```python
from build123d import *

# Parameters (mm, degrees)
BOSS_EXTRUDE1_DEPTH       = 25
F_1_0MM_DOWEL_HOLE1_D     = 10
F_1_0MM_DOWEL_HOLE1_DEPTH = 25
M8X1_0_TAPPED_HOLE1_D     = 7
M8X1_0_TAPPED_HOLE1_DEPTH = 15


# Read off the part's stored shape, not the designer's step: CSK for M6 Flat Head Machine Screw1
with BuildPart() as part:
    # Sketch1 → Boss-Extrude1 (new, symmetric)
    with BuildSketch(Plane.XY):
        Polygon((0, 0), (0, 97), (-45, 97), (-45, 84), (-39, 84), (-39, 90), (-32, 90), (-32, 0), align=None)
    extrude(amount=BOSS_EXTRUDE1_DEPTH, both=True)

    # Ø1.0mm Dowel Hole1
    with Locations(Plane.XY.offset(25)):
        with Locations((-16, 45)):
            Hole(F_1_0MM_DOWEL_HOLE1_D / 2, depth=F_1_0MM_DOWEL_HOLE1_DEPTH)

    # M8x1.0 Tapped Hole1
    with Locations(Plane(origin=(0, 0, 0), x_dir=(-1, 0, 0), z_dir=(0, -1, 0))):
        with Locations((7, 0), (25, 0)):
            Hole(M8X1_0_TAPPED_HOLE1_D / 2, depth=M8X1_0_TAPPED_HOLE1_DEPTH)

    # CSK for M6 Flat Head Machine Screw1 outl → CSK for M6 Flat Head Machine Screw1 (revolve, cut)
    with BuildSketch(Plane(origin=(0, 45, 9), x_dir=(0, 1, 0), z_dir=(0, 0, -1))):
        Polygon((0, -12.244302381), (3.3, -12.244302381), (3.3, -3), (6.3, 0), (0, 0), align=None)
    revolve(axis=Axis((0, 45, 9), (1, 0, 0)), mode=Mode.SUBTRACT)


solid = part.part
```
For this review, take the finished solid that the model builds, in its own axes (mm). A direction names the side the tool comes from. Round coordinates to 2 decimals unless told otherwise and drop trailing zeros. Write each loop counter-clockwise with the first axis right and the second up, starting at its lowest first coordinate (ties: lowest second). Pieces come first, ordered by that corner, then holes.
1) Mouldability with a two-part tool opening along Z and no side actions: class faces 1 (the face through (-25, 15, 0)), 2 (the face through (-16, 45, 0)), 3 (the face through (-7, 15, 0)), 4 (the face through (-32, 46, 0)) as +Z half, -Z half, draft (parallel to the pull), parting line (faces both ways), or undercut.
Answer below:
face 1: undercut
face 2: +Z half
face 3: undercut
face 4: draft
2) Take a section at A-A on y = 45. Give the boundary of the cut face in (x, z), then the cut area to 3 significant figures.
Answer below:
outline: (-32, -25) - (0, -25) - (0, 2.7) - (-3, 5.7) - (-11, 5.7) - (-11, 0) - (-21, 0) - (-21, 25) - (-32, 25) - close; (-11, 12.3) - (-3, 12.3) - (0, 15.3) - (0, 25) - (-11, 25) - close
area: 1,270 mm2
3) Insertion check: pin 1 Ø7.5 at (x, z) = (-36.5, 8.5) entering from -Y; pin 2 Ø3 at (y, z) = (68, 10.5) entering from -X; pin 3 Ø2 at (x, z) = (-25, 0) entering from -Y; pin 4 Ø6 at (x, y) = (-36.5, 73.5) entering from +Z. Each pin has a flat end and moves straight along its axis. Give the tip position at first contact, or say it passes through.
Answer below:
pin 1: stops at y = 84
pin 2: stops at x = -32
pin 3: stops at y = 15
pin 4: passes through
4) Take a section at B-B on x = -7. Give the boundary of the cut face in (y, z), then the cut area to 3 significant figures.
Answer below:
outline: (0, -25) - (97, -25) - (97, 25) - (0, 25) - (0, 3.5) - (15, 3.5) - (15, -3.5) - (0, -3.5) - close; hole circle Ø6.6 at (45, 9)
area: 4,710 mm2
5) Take a section at D-D on x = -19.5. Give the boundary of the cut face in (y, z), then the cut area to 3 significant figures.
Answer below:
outline: (0, -25) - (97, -25) - (97, 25) - (48.57, 25) - (48.57, 0) - (41.43, 0) - (41.43, 25) - (0, 25) - close
area: 4,670 mm2
6) Take a section at C-C on z = -15.5. Give the boundary of the cut face in (x, y).
Answer below:
outline: (-45, 84) - (-39, 84) - (-39, 90) - (-32, 90) - (-32, 0) - (0, 0) - (0, 97) - (-45, 97) - close
7) For line 1 along Z through (x, y) = (-9, 45); line 2 along Z through (x, y) = (-7, 9); line 3 along Y through (x, z) = (-5, 9), list the stretches that pass through material, from the lowest coordinate up.
Answer below:
line 1: z = -25 to 5.7, 12.3 to 25
line 2: z = -25 to -3.5, 3.5 to 25
line 3: y = 0 to 41.7, 48.3 to 97
8) Machinability: for faces 5 (the face through (-39, 87, 0)), 6 (the face through (-42, 84, 0)), 7 (the face through (-10.497, 7.605, -0.154)), 8 (the face through (-7.56, 44.28, 5.78)), which of the approach directions +Z, -Z, +X, -X, +Y, -Y give a long, thin tool a straight path to every point of the face, cutting with its end or side? Answer none if there is none.
Answer below:
face 5: +Z, -Z, -Y
face 6: +Z, -Z, -X, -Y
face 7: -Y
face 8: +X
